from build123d import *

# Parameters (mm, degrees)
F0_R     = 12.5
F1_DEPTH = 6
F2_R     = 22
F3_DEPTH = 36
F4_R     = 13
F5_DEPTH = 34


with BuildPart() as f1:
    # F0 (on Top) → F1 (new body)
    with BuildSketch(Plane.XY):
        Circle(F0_R)
    extrude(amount=F1_DEPTH)

    # F2 (on face) → F3 (join)
    with BuildSketch(Plane(origin=(0, 0, 0), x_dir=(1, 0, 0), z_dir=(0, 0, -1))):
        Circle(F2_R)
    extrude(amount=F3_DEPTH)

    # F4 (on face) → F5 (cut)
    with BuildSketch(Plane(origin=(0, 0, -36), x_dir=(1, 0, 0), z_dir=(0, 0, -1))):
        Circle(F4_R)
    extrude(amount=-F5_DEPTH, mode=Mode.SUBTRACT)


solid = f1.part
Geometry check sheet. Reference: the model listing, model coordinates, mm. A direction names the side the tool comes from. Give positions to 0.01 mm unless a question says otherwise; leave off trailing zeros. Loops run counter-clockwise (first coordinate to the right, second up) from the corner with the lowest first, then second, coordinate; pieces in that order, holes last. Notation, with made-up numbers: M -31.5,40.5 L 12.5,40.5 A14 cw 12.5,65.5 Z; hole C 69.25,20 d1. An arc over 180 degrees is marked long. Answer as a JSON object with one key per item and string values. Group by question number.
Item 1: Material ranges on L1, parallel to X at y = 0, z = -9; L2, parallel to Z at x = -18, y = -8.5, recorded low to high.
Item 2: Gauge pin test, flat ends, axial feed: pin 1 (4 mm diameter, centred on x = 8.5, z = -29, fed in from +Y); pin 2 (12 mm diameter, centred on y = 9, z = -20.5, fed in from -X); pin 3 (1 mm diameter, centred on x = 10, z = -14.5, fed in from -Y). Record the tip position at first contact, or that the pin passes through.
Item 3: Sectioned sample at A-A on y = 0. Record the boundary of the cut face in (x, z).
Item 4: Sectioned sample at B-B on z = -8.5. Record the boundary of the cut face in (x, y).
Item 5: Mould release check, pull along X, two halves, no side actions. Record for faces 1 (the cylindrical face through (-4.769, 21.477, -17.748)), 2 (the flat face through (9, 9, 0)), 3 (the flat face through (0, 0, -2)): pulls with the +X half, pulls with the -X half, needs draft (parallel to the pull), parting line crosses it, or undercut.
Item 6: Sectioned sample at D-D on z = 2. Record the boundary of the cut face in (x, y).
Item 7: Access from +Z, -Z, +X, -X, +Y, -Y to the whole of each face (thin tool, end or side, straight path). Record for faces 4 (the flat face through (9.5, 9.5, -36)), 5 (the cylindrical face through (-10.316, 7.91, -19.238)), 6 (the cylindrical face through (11.923, 3.755, 2.958)).
Findings below:
{
 "1": {"L1": "-22 to -13, 13 to 22", "L2": "-36 to 0"},
 "2": {"pin 1": "y = 21.02", "pin 2": "x = -21.79", "pin 3": "y = -19.84"},
 "3": {"outline": "M -22,-36 L -13,-36 L -13,-2 L 13,-2 L 13,-36 L 22,-36 L 22,0 L 12.5,0 L 12.5,6 L -12.5,6 L -12.5,0 L -22,0 Z"},
 "4": {"outline": "C 0,0 d44; hole C 0,0 d26"},
 "5": {"face 1": "parting line crosses it", "face 2": "needs draft", "face 3": "undercut"},
 "6": {"outline": "C 0,0 d25"},
 "7": {"face 4": "-Z, +X, -X, +Y, -Y", "face 5": "-Z", "face 6": "+Z"}
}
